Geometry: final body of the model. Coordinates: model frame, mm. Give positions to 0.01 mm unless a question says otherwise; leave off trailing zeros. Write each loop counter-clockwise with the first axis right and the second up, starting at its lowest first coordinate (ties: lowest second). Pieces come first, ordered by that corner, then holes. Notation, with made-up numbers: M 16.25,65.25 L 51.25,65.25 A17 ccw 51.25,82.25 Z; hole C -2.5,79.25 d7. An arc over 180 degrees is marked long. Use one line per item in the form item = value. Start each with the question number.
Item 1: Material intervals for line 1 along X through (y, z) = (1.4, 0); line 2 along Z through (x, y) = (-20, 4.2); line 3 along X through (y, z) = (3.2, 6.5), sorted ascending. Write a range as from..to.
Item 2: Section query A-A on y = 1.6. Return loops of the section in (x, z).
Item 3: Section query B-B on z = -64. Return loops of the section in (x, y).
Item 4: Section query C-C on x = 80. Return loops of the section in (y, z), then the cut area to 3 significant figures.
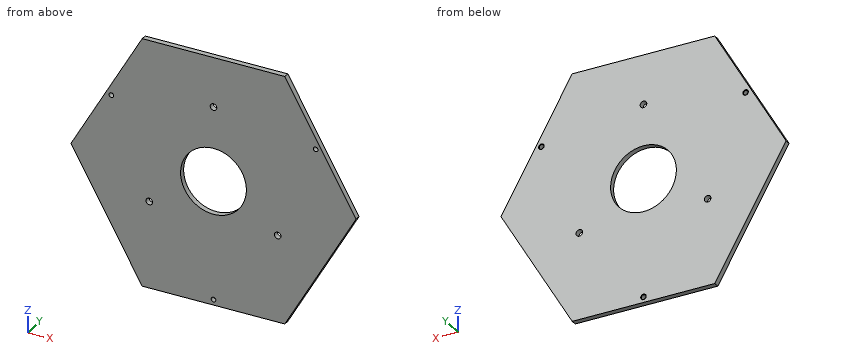
from build123d import *

# Parameters (mm, degrees)
EXTRUDE_1_DEPTH              = 5
SKETCH_2_R                   = 30
CUT_EXTRUDE_1_DEPTH          = 5
SKETCH_3_R                   = 3
CUT_EXTRUDE_2_DEPTH          = 5
HOLE_WIZARD_M5_3_D           = 4.2
HOLE_WIZARD_M5_3_CSINK_D     = 5.05
HOLE_WIZARD_M5_3_CSINK_ANGLE = 90


with BuildPart() as part:
    # 草图1 → 凸台-拉伸1 (new body)
    with BuildSketch(Plane(origin=(0, 0, 0), x_dir=(1, 0, 0), z_dir=(0, 1, 0))):
        Polygon((130, 0), (65, 112.583302492), (-65, 112.583302492), (-130, 0), (-65, -112.583302492), (65, -112.583302492), align=None)
    extrude(amount=EXTRUDE_1_DEPTH)

    # 草图2 → 切除-拉伸1 (cut)
    with BuildSketch(Plane(origin=(0, 5, 0), x_dir=(1, 0, 0), z_dir=(0, 1, 0))):
        with Locations(Location((0, 0, 0), (0, 0, 270))):
            Circle(SKETCH_2_R)
    extrude(amount=-CUT_EXTRUDE_1_DEPTH, mode=Mode.SUBTRACT)

    # 草图3 → 切除-拉伸2 (cut)
    with BuildSketch(Plane(origin=(0, 5, 0), x_dir=(1, 0, 0), z_dir=(0, 1, 0))):
        with Locations(Location((-58.52885683, 33.791651246, 0), (0, 0, 270))):
            Circle(SKETCH_3_R)
        with Locations(Location((58.52885683, 33.791651246, 0), (0, 0, 270))):
            Circle(SKETCH_3_R)
        with Locations(Location((0, -67.583302492, 0), (0, 0, 270))):
            Circle(SKETCH_3_R)
    extrude(amount=-CUT_EXTRUDE_2_DEPTH, mode=Mode.SUBTRACT)

    # M5 螺纹孔3 (through all)
    with Locations(Plane(origin=(0, 5, 0), x_dir=(1, 0, 0), z_dir=(0, 1, 0))):
        with Locations((0, 107.533302492), (-93.126571711, -53.766651246), (93.126571711, -53.766651246)):
            CounterSinkHole(HOLE_WIZARD_M5_3_D / 2, HOLE_WIZARD_M5_3_CSINK_D / 2, counter_sink_angle=HOLE_WIZARD_M5_3_CSINK_ANGLE)


solid = part.part
Answer sheet:
q1.line_1 = -130..-30, 30..130
q1.line_2 = -112.58..-22.36, 22.36..112.58
q1.line_3 = -126.25..-29.29, 29.29..126.25
q2.outline = M -130,0 L -65,-112.58 L 65,-112.58 L 130,0 L 65,112.58 L -65,112.58 Z; hole C -93.13,53.77 d4.2; hole C -58.53,-33.79 d6; hole C 0,0 d60; hole C 0,67.58 d6; hole C 0,-107.53 d4.2; hole C 58.53,-33.79 d6; hole C 93.13,53.77 d4.2
q3.outline = M -93.05,0 L 93.05,0 L 93.05,5 L -93.05,5 Z
q4.outline = M 0,-86.6 L 5,-86.6 L 5,86.6 L 0,86.6 Z
q4.area = 866 mm2
